```python
from build123d import *

# Parameters (mm, degrees)
SKETCH1_R               = 1.5
BOSS_EXTRUDE1_DEPTH     = 3
SKETCH2_R               = 1.5
CUT_EXTRUDE1_DEPTH      = 124.30125084
MIRROR2_COPY_1_SKETCH_R = 1.5
MIRROR2_COPY_1_DEPTH    = 124.30125084


with BuildPart() as part:
    # Sketch1 → Boss-Extrude1 (new body)
    with BuildSketch(Plane(origin=(0, 0, 0), x_dir=(1, 0, 0), z_dir=(0, 1, 0))):
        with BuildLine():
            Line((-89.116425142, 53.107925476), (-18, 14.012636522))
            Line((-18, 14.012636522), (-18, -14.012636522))
            Line((-18, -14.012636522), (-89.116425142, -53.107925476))
            ThreePointArc((-89.116425142, -53.107925476), (-94.245861402, -70.762638264), (-76.591148614, -75.892074524))
            Line((-76.591148614, -75.892074524), (-18, -43.682386248))
            Line((-18, -43.682386248), (-18, -73.682386248))
            Line((-18, -73.682386248), (18, -73.682386248))
            Line((18, -73.682386248), (18, -43.682386248))
            Line((18, -43.682386248), (76.591148614, -75.892074524))
            ThreePointArc((76.591148614, -75.892074524), (94.245861402, -70.762638264), (89.116425142, -53.107925476))
            Line((89.116425142, -53.107925476), (18, -14.012636522))
            Line((18, -14.012636522), (18, 14.012636522))
            Line((18, 14.012636522), (89.116425142, 53.107925476))
            ThreePointArc((89.116425142, 53.107925476), (94.245861402, 70.762638264), (76.591148614, 75.892074524))
            Line((76.591148614, 75.892074524), (18, 43.682386248))
            Line((18, 43.682386248), (18, 73.682386248))
            Line((18, 73.682386248), (-18, 73.682386248))
            Line((-18, 73.682386248), (-18, 43.682386248))
            Line((-18, 43.682386248), (-76.591148614, 75.892074524))
            ThreePointArc((-76.591148614, 75.892074524), (-94.245861402, 70.762638264), (-89.116425142, 53.107925476))
        make_face()
        with Locations(Location((-15.25, 15.25, 0), (0, 0, 270))):
            Circle(SKETCH1_R, mode=Mode.SUBTRACT)
        with Locations(Location((-15.25, 67.75, 0), (0, 0, 270))):
            Circle(SKETCH1_R, mode=Mode.SUBTRACT)
        with Locations(Location((-15.25, -60.25, 0), (0, 0, 270))):
            Circle(SKETCH1_R, mode=Mode.SUBTRACT)
        with Locations(Location((15.25, 67.75, 0), (0, 0, 270))):
            Circle(SKETCH1_R, mode=Mode.SUBTRACT)
        with Locations(Location((15.25, 15.25, 0), (0, 0, 270))):
            Circle(SKETCH1_R, mode=Mode.SUBTRACT)
        with Locations(Location((15.25, -15.25, 0), (0, 0, 270))):
            Circle(SKETCH1_R, mode=Mode.SUBTRACT)
        with Locations(Location((-15.25, -15.25, 0), (0, 0, 270))):
            Circle(SKETCH1_R, mode=Mode.SUBTRACT)
        with Locations(Location((15.25, -60.25, 0), (0, 0, 270))):
            Circle(SKETCH1_R, mode=Mode.SUBTRACT)
    extrude(amount=BOSS_EXTRUDE1_DEPTH)

    # Sketch2 → Cut-Extrude1 (cut, through all)
    with BuildSketch(Plane(origin=(0, 3, 0), x_dir=(1, 0, 0), z_dir=(0, 1, 0))):
        with Locations(Location((-85.085823286, 72.182318236, 0), (0, 0, 270))):
            Circle(SKETCH2_R)
        with Locations(Location((-75.171468642, 66.732036408, 0), (0, 0, 270))):
            Circle(SKETCH2_R)
        with Locations(Location((-80.62175047, 56.817681764, 0), (0, 0, 90))):
            Circle(SKETCH2_R)
        with Locations(Location((-90.536105113, 62.267963592, 0), (0, 0, 90))):
            Circle(SKETCH2_R)
    cut_extrude1 = extrude(amount=-CUT_EXTRUDE1_DEPTH, mode=Mode.SUBTRACT)

    # Mirror1: Cut-Extrude1 across plane
    add(cut_extrude1.mirror(Plane.XY), mode=Mode.SUBTRACT)

    # Mirror2: Cut-Extrude1 across plane
    add(cut_extrude1.mirror(Plane(origin=(0, 0, 0), x_dir=(0, 0, 1), z_dir=(1, 0, 0))), mode=Mode.SUBTRACT)

    # Mirror2 copy 1 sketch → Mirror2 copy 1 (cut, through all)
    with BuildSketch(Plane(origin=(0, 3, 0), x_dir=(-1, 0, 0), z_dir=(0, 1, 0))):
        with Locations(Location((-85.085823286, 72.182318236, 0), (0, 0, 270))):
            Circle(MIRROR2_COPY_1_SKETCH_R)
        with Locations(Location((-75.171468642, 66.732036408, 0), (0, 0, 270))):
            Circle(MIRROR2_COPY_1_SKETCH_R)
        with Locations(Location((-80.62175047, 56.817681764, 0), (0, 0, 90))):
            Circle(MIRROR2_COPY_1_SKETCH_R)
        with Locations(Location((-90.536105113, 62.267963592, 0), (0, 0, 90))):
            Circle(MIRROR2_COPY_1_SKETCH_R)
    extrude(amount=-MIRROR2_COPY_1_DEPTH, mode=Mode.SUBTRACT)


solid = part.part
```
Check sheet for the modelled part. Datum: model origin and axes. Units: mm. A direction names the side the tool comes from. Coordinates: 2 decimals unless noted, no trailing zeros. Order: outer loops, then holes, each group sorted by start corner. A loop starts at its lowest first (then second) coordinate and runs counter-clockwise, first axis right, second up. Notation, with made-up numbers: (70, 28) -> (90, 28) arc R26 cw to (90, 51) -> close; hole circle Ø3 at (-19, 12). An arc over 180 degrees is marked (long way). Write each question's results on one line, items separated by ' | '. Start each with the question number.
1) Section check B-B (z = -50). Enter the section's corners in (x, y).
2) Section check C-C (y = 0.9). Count the separate pieces of the cut face and the enclosed holes in it, and give its area (3 significant figures).
3) Draft check along Z on faces 1 (the face through (94.105, 1.479, 71.012)), 2 (the face through (-47.706, 1.479, 60.013)), 3 (the face through (-94.105, 1.479, -71.012)), 4 (the face through (-46.885, 1.479, -59.562)). Enter one of: pulls with the +Z half, pulls with the -Z half, needs draft (parallel to the pull), parting line crosses it, or undercut.
4) Depth check by flat-ended pin: pin 1 (1.5 mm diameter, centred on y = 1, z = 66, fed in from -X). Enter the tip coordinate at first touch or a pass-through.
5) Material ranges on line 1 along Z through (x, y) = (-15.5, 1.8); line 2 along X through (y, z) = (0.95, -64.5); line 3 along X through (y, z) = (0.3, 46), recorded low to high.
6) Section check A-A (x = -32.5). Enter the section's corners in (y, z), and give its area (3 significant figures).
7) Set-up check for faces 5 (the face through (53.06, 1.479, -33.287)), 6 (the face through (47.706, 1.479, -60.013)), 7 (the face through (-54.056, 1.479, -33.834)): record each of +Z, -Z, +X, -X, +Y, -Y from which the full face is reachable in a straight line by a thin tool's end or side.
8) Section check D-D (x = 1). Enter the section's corners in (y, z).
Checked values:
1) outline: (-83.46, 0) -> (-29.49, 0) -> (-29.49, 3) -> (-83.46, 3) -> close; (-18, 0) -> (18, 0) -> (18, 3) -> (-18, 3) -> close; (29.49, 0) -> (83.46, 0) -> (83.46, 3) -> (29.49, 3) -> close
2) separate pieces: 1 | enclosed holes: 24 | area: 13,900 mm²
3) face 1: undercut | face 2: pulls with the +Z half | face 3: undercut | face 4: pulls with the -Z half
4) pin 1: x = -95.83
5) line 1: -73.68 to -69.23, -66.27 to -16.73, -13.77 to 13.77, 16.73 to 58.77, 61.73 to 73.68 | line 2: -95.85 to -55.87, -18 to 18, 55.87 to 95.85 | line 3: -76.19 to -22.22, -18 to 18, 22.22 to 76.19
6) outline: (0, -51.65) -> (3, -51.65) -> (3, -21.98) -> (0, -21.98) -> close; (0, 21.98) -> (3, 21.98) -> (3, 51.65) -> (0, 51.65) -> close | area: 178 mm²
7) face 5: +X, +Y, -Y | face 6: -Z, +Y, -Y | face 7: -X, +Y, -Y
8) outline: (0, -73.68) -> (3, -73.68) -> (3, 73.68) -> (0, 73.68) -> close
